For this review, take the finished solid that the model builds, in its own axes (mm). Face numbers are marked on the shaded views. A direction names the side the tool comes from. Round coordinates to 2 decimals unless told otherwise and drop trailing zeros. Loops run counter-clockwise (first coordinate to the right, second up) from the corner with the lowest first, then second, coordinate; pieces in that order, holes last. Notation, with made-up numbers: (-27.75, 53) -> (0.25, 53) arc R34 ccw to (0.25, 87) -> close; hole circle Ø8 at (43, 84.25). An arc over 180 degrees is marked (long way). Write each question's results on one line, items separated by ' | '.
```python
from build123d import *

# Parameters (mm, degrees)
BOSS_EXTRUDE1_DEPTH      = 3
SKETCH2_R                = 1.5
BOSS_EXTRUDE2_DEPTH      = 2.5
BOSS_EXTRUDE2_DEPTH_BACK = 22.3
SKETCH3_W                = 2.5
SKETCH3_H                = 20.733799839
CUT_EXTRUDE1_DEPTH       = 4
CUT_EXTRUDE1_DEPTH_BACK  = 1
BOSS_EXTRUDE3_START      = -0.5
BOSS_EXTRUDE3_DEPTH      = 5.8
FILLET1_R                = 0.5
FILLET1_OF_MIRROR1_R     = 0.5
CUT_EXTRUDE2_DEPTH       = 23.3000001
SKETCH8_W                = 15
SKETCH8_H                = 4.3
CUT_EXTRUDE3_DEPTH       = 1.5
FILLET2_R                = 0.5
FILLET3_R                = 1


with BuildPart() as part:
    # Sketch1 → Boss-Extrude1 (new body)
    with BuildSketch(Plane.XY):
        with BuildLine():
            Line((3.2, 25.3), (3.2, 12.05))
            ThreePointArc((3.2, 12.05), (4.45, 10.8), (5.7, 12.05))
            Line((5.7, 12.05), (5.7, 25.3))
            Line((5.7, 25.3), (14.1, 25.3))
            Line((14.1, 25.3), (14.1, 12.05))
            ThreePointArc((14.1, 12.05), (15.35, 10.8), (16.6, 12.05))
            Line((16.6, 12.05), (16.6, 25.3))
            Line((16.6, 25.3), (19.8, 25.3))
            Line((19.8, 25.3), (19.8, 0))
            Line((19.8, 0), (0, 0))
            Line((0, 0), (0, 25.3))
            Line((0, 25.3), (3.2, 25.3))
        make_face()
    extrude(amount=BOSS_EXTRUDE1_DEPTH)

    # Sketch2 → Boss-Extrude2 (add, two sides)
    with BuildSketch(Plane(origin=(19.8, 0, 0), x_dir=(0, 0, -1), z_dir=(1, 0, 0))) as boss_extrude2_sk:
        with Locations((-1.5, 25.3)):
            Circle(SKETCH2_R)
    extrude(amount=BOSS_EXTRUDE2_DEPTH)
    extrude(boss_extrude2_sk.sketch, amount=-BOSS_EXTRUDE2_DEPTH_BACK)

    # Sketch3 → Cut-Extrude1 (cut, two sides)
    with BuildSketch(Plane.XY) as cut_extrude1_sk:
        with Locations((4.45, 22.41689992)):
            Rectangle(SKETCH3_W, SKETCH3_H)
        with Locations((15.35, 22.41689992)):
            Rectangle(SKETCH3_W, SKETCH3_H)
    extrude(amount=CUT_EXTRUDE1_DEPTH, mode=Mode.SUBTRACT)
    extrude(cut_extrude1_sk.sketch, amount=-CUT_EXTRUDE1_DEPTH_BACK, mode=Mode.SUBTRACT)

    # Sketch5 → Boss-Extrude3 (add)
    with BuildSketch(Plane(origin=(0, 26.8, 0), x_dir=(1, 0, 0), z_dir=(0, 1, 0)).offset(BOSS_EXTRUDE3_START)):
        with BuildLine():
            Line((0, -0.75), (0, -2.25))
            ThreePointArc((0, -2.25), (-0.75, -1.5), (0, -0.75))
        make_face()
    boss_extrude3 = extrude(amount=-BOSS_EXTRUDE3_DEPTH)

    # Fillet1
    fillet1_edges = [part.edges().sort_by_distance(p)[0] for p in [
        (-0.75, 20.5, 1.5),
    ]]
    fillet(fillet1_edges, radius=FILLET1_R)

    # Mirror1: Boss-Extrude3 across plane
    add(boss_extrude3.mirror(Plane.ZY.offset(-9.9)))

    # Fillet1 of Mirror1
    fillet1_of_mirror1_edges = [part.edges().sort_by_distance(p)[0] for p in [
        (20.55, 20.5, 1.5),
    ]]
    fillet(fillet1_of_mirror1_edges, radius=FILLET1_OF_MIRROR1_R)

    # Sketch6 → Cut-Extrude2 (cut, through all)
    with BuildSketch(Plane.ZY):
        Polygon((0, 0), (3, 2), (3, -2.592158126), (0, -2.592158126), align=None)
    extrude(amount=-CUT_EXTRUDE2_DEPTH, mode=Mode.SUBTRACT)

    # Sketch8 → Cut-Extrude3 (cut)
    with BuildSketch(Plane(origin=(0, -0.802775638, 1.499997875), x_dir=(-1, 0, 0), z_dir=(0, 0.471858445, -0.881674321))):
        with Locations((-9.9, 3.178923977)):
            Rectangle(SKETCH8_W, SKETCH8_H)
    extrude(amount=CUT_EXTRUDE3_DEPTH, mode=Mode.SUBTRACT)

    # Fillet2
    fillet2_edges = [part.edges().sort_by_distance(p)[0] for p in [
        (-2.5, 25.3, 3),
        (22.3, 25.3, 3),
    ]]
    fillet(fillet2_edges, radius=FILLET2_R)

    # Fillet3
    fillet3_edges = [part.edges().sort_by_distance(p)[0] for p in [
        (19.8, 1, 1.5),
        (0, 1, 1.5),
    ]]
    fillet(fillet3_edges, radius=FILLET3_R)


solid = part.part
```
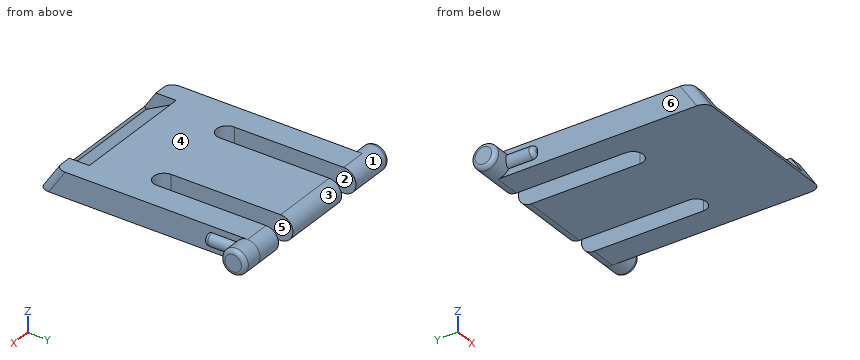
1. Consider section B-B (x = 4.45). State the section outline as (y, z) points.
Values found:
outline: (0, 0) -> (10.8, 0) -> (10.8, 3) -> (4.44, 3) -> (4.6, 2.69) -> (0.81, 0.66) -> (0.65, 0.97) -> close
2. Consider section D-D (x = 8.75). State the section outline as (y, z) points, plus the area to 3 significant figures.
Values found:
outline: (0, 0) -> (25.3, 0) arc R1.5 ccw to (25.3, 3) -> (4.44, 3) -> (4.6, 2.69) -> (0.81, 0.66) -> (0.65, 0.97) -> close | area: 72.5 mm2
3. To check wall thickness, follow probe 1 along X at (y, z) = (24.75, 1.8); probe 2 along X at (y, z) = (19.75, 1.5); probe 3 along X at (y, z) = (4, 2.15). State the ranges of each line that lie inside material, in increasing order.
Values found:
probe 1: x = -2.5 to 3.2, 5.7 to 14.1, 16.6 to 22.3 | probe 2: x = 0 to 3.2, 5.7 to 14.1, 16.6 to 19.8 | probe 3: x = 0 to 19.8
4. Draft analysis for pull direction X (two halves, no side actions). For the marked faces 4, 5 and 6, state which applies: released by +X, released by -X, zero draft, split by the parting line, or undercut.
Values found:
face 4: zero draft | face 5: undercut | face 6: released by -X
5. For pin 1 (1.5 mm diameter, centred on y = 20, z = 1.5, fed in from +X); pin 2 (0.9 mm diameter, centred on y = 12, z = 2, fed in from +X); pin 3 (1.2 mm diameter, centred on y = 3.5, z = 1.5, fed in from -X), all flat-tipped, find the tip position at first contact; note any pin that passes through.
Values found:
pin 1: stops at x = 20.48 | pin 2: stops at x = 19.8 | pin 3: stops at x = 0
6. Consider section A-A (y = 11.5). State the section outline as (x, z) points.
Values found:
outline: (0, 0) -> (3.33, 0) -> (3.33, 3) -> (0, 3) -> close; (5.57, 0) -> (14.23, 0) -> (14.23, 3) -> (5.57, 3) -> close; (16.47, 0) -> (19.8, 0) -> (19.8, 3) -> (16.47, 3) -> close
7. Consider section C-C (y = 5.5). State the section outline as (x, z) points, plus the area to 3 significant figures.
Values found:
outline: (0, 0) -> (19.8, 0) -> (19.8, 3) -> (0, 3) -> close | area: 59.4 mm2
8. Tool access review of the marked faces 1, 2 and 3: name each direction out of +Z, -Z, +X, -X, +Y, -Y from which nothing blocks a thin tool from reaching the whole face with its end or side.
Values found:
face 1: -X | face 2: +Z, -Z, +Y | face 3: +X, -X, +Y
